Read the model definition and answer for the solid it produces. Units are mm, in the model's axes. Face numbers are marked on the shaded views. A direction names the side the tool comes from. Coordinates: 2 decimals unless noted, no trailing zeros. Order: outer loops, then holes, each group sorted by start corner. A loop starts at its lowest first (then second) coordinate and runs counter-clockwise, first axis right, second up. Notation, with made-up numbers: M 21.5,79 L 74.5,79 A26 ccw 74.5,117 Z; hole C -22.5,-2.75 d6. An arc over 180 degrees is marked long. Put each result on its own line as item: value.
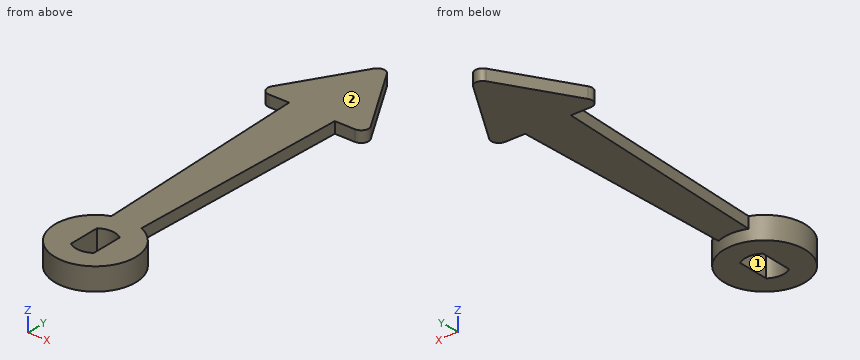
from build123d import *

# Parameters (mm, degrees)
F0_R     = 5.4
F1_DEPTH = 1.5
F3_DEPTH = 1.5
F6_DEPTH = 1.5
F7_R     = 1


with BuildPart() as f1:
    # F0 (on Top) → F1 (new body, symmetric)
    with BuildSketch(Plane.XY):
        Circle(F0_R)
        with BuildLine():
            ThreePointArc((1.525, 2.105796), (2.315707, 1.182159), (2.6, 0))
            ThreePointArc((2.6, 0), (2.315707, -1.182159), (1.525, -2.105796))
            ThreePointArc((1.525, -2.105796), (0, -2.6), (-1.525, -2.105796))
            ThreePointArc((-1.525, -2.105796), (-2.6, 0), (-1.525, 2.105796))
            ThreePointArc((-1.525, 2.105796), (0, 2.6), (1.525, 2.105796))
        make_face(mode=Mode.SUBTRACT)
        with BuildLine():
            Line((-1.525, -2.105796), (-1.525, 2.105796))
            ThreePointArc((-1.525, 2.105796), (-2.6, 0), (-1.525, -2.105796))
        make_face()
        with BuildLine():
            ThreePointArc((1.525, -2.105796), (2.315707, -1.182159), (2.6, 0))
            ThreePointArc((2.6, 0), (2.315707, 1.182159), (1.525, 2.105796))
            Line((1.525, 2.105796), (1.525, -2.105796))
        make_face()
    extrude(amount=F1_DEPTH, both=True)

    # F2 (on Top) → F3 (join, through all)
    with BuildSketch(Plane.XY):
        Polygon((-2, 5.015974), (0, 5.015974), (2, 5.015974), (3.047065, 35), (0, 35), (-3.047065, 35), align=None)
    extrude(amount=F3_DEPTH)

    # F5 (on Top) → F6 (join, through all)
    with BuildSketch(Plane.XY):
        Polygon((0, 47.5), (-7.5, 35), (7.5, 35), align=None)
    extrude(amount=F6_DEPTH)

    # F7
    f7_edges = [f1.edges().sort_by_distance(p)[0] for p in [
        (0, 47.5, 0.75),
        (-7.5, 35, 0.75),
        (7.5, 35, 0.75),
    ]]
    fillet(f7_edges, radius=F7_R)


solid = f1.part
Q1. A tool of negligible diameter and unlimited length cuts with its end or side. For the marked faces 1 and 2, from which of +Z, -Z, +X, -X, +Y, -Y can it reach the whole face along a straight path? Write none if from no direction.
Answers below:
face 1: +Z, -Z
face 2: +Z, +X, -X, +Y, -Y
Q2. Find section C-C on z = -0.65. Write down the section's boundary in (x, y) (3 decimals), plus the area to 3 significant figures.
Answers below:
outline: C 0,0 d10.8; hole M -1.525,-2.106 A2.6 ccw 1.525,-2.106 L 1.525,2.106 A2.6 ccw -1.525,2.106 Z
area: 76.7 mm^2
Q3. Find section A-A on x = 0. Write down the section's boundary in (y, z).
Answers below:
outline: M -5.4,-1.5 L -2.6,-1.5 L -2.6,1.5 L -5.4,1.5 Z; M 2.6,-1.5 L 5.4,-1.5 L 5.4,0 L 46.56,0 L 46.56,1.5 L 2.6,1.5 Z
Q4. Find section B-B on y = 0. Write down the section's boundary in (x, z) (3 decimals).
Answers below:
outline: M -5.4,-1.5 L -1.525,-1.5 L -1.525,1.5 L -5.4,1.5 Z; M 1.525,-1.5 L 5.4,-1.5 L 5.4,1.5 L 1.525,1.5 Z
Q5. Consider line 1 along Z through (x, y) = (2, 8); line 2 along Y through (x, z) = (0.25, -0.5); line 3 along X through (y, z) = (0.5, -0.05) (3 decimals). Determine where each line is inside the solid, lowest interval first.
Answers below:
line 1: z = 0 to 1.5
line 2: y = -5.39 to -2.59, 2.59 to 5.39
line 3: x = -5.377 to -1.525, 1.525 to 5.377
Q6. Given pin 1 (0.8 mm diameter, centred on x = -4.5, z = 1, fed in from -Y); pin 2 (0.9 mm diameter, centred on y = 0, z = 0.5, fed in from +X); pin 3 (2 mm diameter, centred on x = -4, y = 18.5, fed in from +Z); pin 4 (1.2 mm diameter, centred on x = 4.5, z = 0.5, fed in from -Y), each flat-ended and moving along its own axis, determine where each tip first touches the part or whether it passes through.
Answers below:
pin 1: stops at y = -3.51
pin 2: stops at x = 5.4
pin 3: passes through
pin 4: stops at y = -3.73
Q7. Find section D-D on y = 41.5. Write down the section's boundary in (x, z).
Answers below:
outline: M -3.6,0 L 3.6,0 L 3.6,1.5 L -3.6,1.5 Z
